Check sheet for the modelled part. Datum: model origin and axes. Units: mm. Face numbers are marked on the shaded views. Give positions to 0.01 mm unless a question says otherwise; leave off trailing zeros. Order: outer loops, then holes, each group sorted by start corner. A loop starts at its lowest first (then second) coordinate and runs counter-clockwise, first axis right, second up.
```python
from build123d import *

# Parameters (mm, degrees)
MODEL_R                  = 1.8
MODEL_R_2                = 3
RESSALTO_EXTRUS_O1_DEPTH = 6


with BuildPart() as part:
    # Model → Ressalto-extrusão1 (new body)
    with BuildSketch(Plane.XY):
        with BuildLine():
            Line((57.173673193, 108.36959926), (33.573673193, 108.36959926))
            Line((33.573673193, 108.36959926), (33.573673193, 5.671329379))
            Line((33.573673193, 5.671329379), (38.573673193, 5.671329379))
            Line((38.573673193, 5.671329379), (57.173673193, 59.671329379))
            Line((57.173673193, 59.671329379), (57.173673193, 76.071329379))
            Line((57.173673193, 76.071329379), (53.673673193, 76.071329379))
            ThreePointArc((53.673673193, 76.071329379), (47.673673193, 82.071329379), (53.673673193, 88.071329379))
            Line((53.673673193, 88.071329379), (57.173673193, 88.071329379))
            Line((57.173673193, 88.071329379), (57.173673193, 108.36959926))
        make_face()
        with Locations((52.673673193, 63.671329379)):
            Circle(MODEL_R, mode=Mode.SUBTRACT)
        with Locations((52.673673193, 99.058930778)):
            Circle(MODEL_R_2, mode=Mode.SUBTRACT)
    extrude(amount=RESSALTO_EXTRUS_O1_DEPTH)


solid = part.part
```
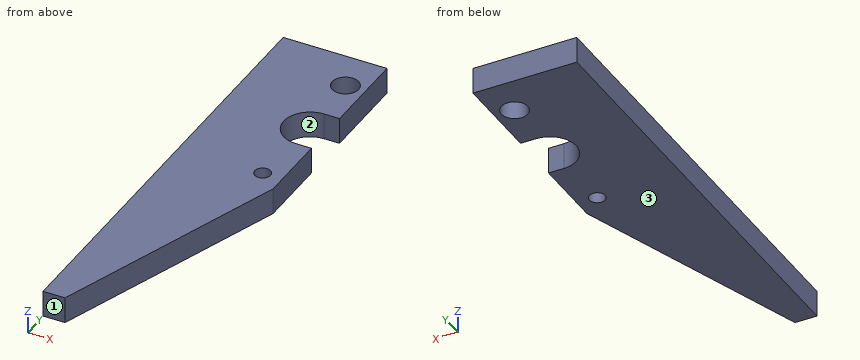
(1) Cross-section at D-D on y = 50.5. Enter the section's corners in (x, z).
Response values:
outline: (33.57, 0) - (54.01, 0) - (54.01, 6) - (33.57, 6) - close
(2) Material ranges on L1, parallel to X at y = 62.5, z = 1.15; L2, parallel to X at y = 80, z = 5.2; L3, parallel to X at y = 24, z = 3.75, recorded low to high.
Response values:
L1: x = 33.57 to 51.31, 54.04 to 57.17
L2: x = 33.57 to 48.04
L3: x = 33.57 to 44.89
(3) Cross-section at A-A on y = 101. Enter the section's corners in (x, z).
Response values:
outline: (33.57, 0) - (50.39, 0) - (50.39, 6) - (33.57, 6) - close; (54.96, 0) - (57.17, 0) - (57.17, 6) - (54.96, 6) - close
(4) Gauge pin test, flat end, axial feed: pin 1 Ø2 at (x, y) = (52.67, 63.67) entering from +Z. Record the tip position at first contact, or that the pin passes through.
Response values:
pin 1: passes through
(5) Release check for a two-part mould opening along Y. For the marked faces 1, 2 and 3 record: released by +Y, released by -Y, zero draft, split by the parting line, or undercut.
Response values:
face 1: released by -Y
face 2: undercut
face 3: zero draft
(6) Cross-section at B-B on z = 2.35. Enter the section's corners in (x, y), then the cut area to 3 significant figures.
Response values:
outline: (33.57, 5.67) - (38.57, 5.67) - (57.17, 59.67) - (57.17, 76.07) - (53.67, 76.07) arc R6 cw to (53.67, 88.07) - (57.17, 88.07) - (57.17, 108.37) - (33.57, 108.37) - close; hole circle Ø6 at (52.67, 99.06); hole circle Ø3.6 at (52.67, 63.67)
area: 1,780 mm2
(7) Cross-section at C-C on x = 46.25. Enter the section's corners in (y, z).
Response values:
outline: (27.96, 0) - (108.37, 0) - (108.37, 6) - (27.96, 6) - close
